Check sheet for the drawn part. Datum: minimum x, y, z corner. Units: mm. Give positions to 0.01 mm unless a question says otherwise; leave off trailing zeros. Loops run counter-clockwise (first coordinate to the right, second up) from the corner with the lowest first, then second, coordinate; pieces in that order, holes last. Notation, with made-up numbers: (76, -2) - (110, -2) arc R15 ccw to (110, 24) - close; hole circle Ø9 at (-7.5, 39). An arc over 180 degrees is marked (long way). Use one line per item in the form item = value.
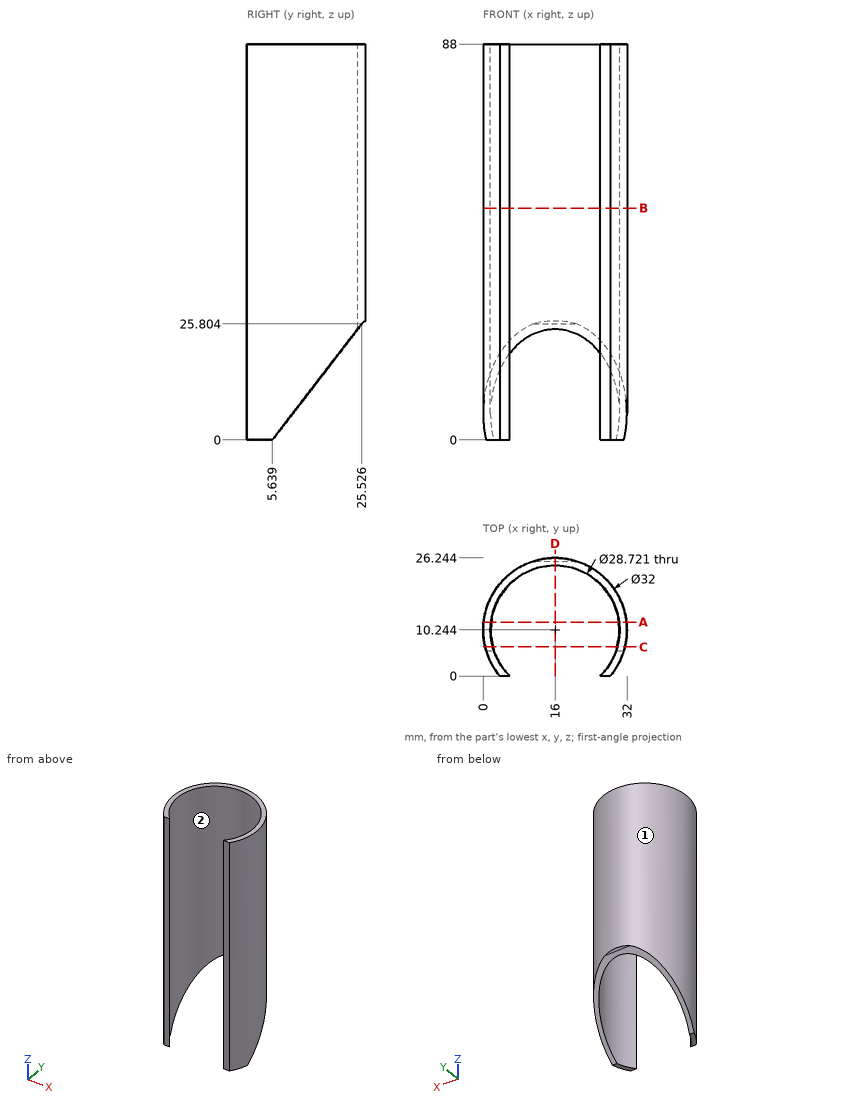
Item 1: Thickness scan on L1, parallel to X at y = 20.5, z = 43; L2, parallel to X at y = 9, z = 70.5; L3, parallel to Y at x = 16, z = 34.5. Record the ranges inside material, lowest first.
Answer block:
L1 = 3.72 to 5.95, 26.05 to 28.28
L2 = 0.05 to 1.69, 30.31 to 31.95
L3 = 24.6 to 26.24
Item 2: Section check D-D on x = 16. Record the boundary of the cut face in (y, z) (1 decimal), then the cut area to 3 significant figures.
Answer block:
outline = (24.6, 24.6) - (25.5, 25.8) - (26.2, 26.4) - (26.2, 88) - (24.6, 88) - close
area = 102 mm2
Item 3: Gauge pin test, flat ends, axial feed: P1, Ø6, axis at y = 12, z = 31, coming from the +X side; P2, Ø3, axis at x = 28, z = 46, coming from the +Y side (1 decimal). Record the tip position at first contact, or that the pin passes through.
Answer block:
P1 = 32
P2 = 22.3
Item 4: Section check A-A on y = 12. Record the boundary of the cut face in (x, z).
Answer block:
outline = (0.1, 8.25) - (1.75, 8.25) - (1.75, 88) - (0.1, 88) - close; (30.25, 8.25) - (31.9, 8.25) - (31.9, 88) - (30.25, 88) - close
Item 5: Section check B-B on z = 51.5. Record the boundary of the cut face in (x, y) (1 decimal), then the cut area to 3 significant figures.
Answer block:
outline = (3.7, 0) - (5.9, 0) arc R14.4 cw (long way) to (26.1, 0) - (28.3, 0) arc R16 ccw (long way) to start
area = 115 mm2
Item 6: Section check C-C on y = 6.5. Record the boundary of the cut face in (x, z) (1 decimal).
Answer block:
outline = (0.4, 1.1) - (2.1, 1.1) - (2.1, 88) - (0.4, 88) - close; (29.9, 1.1) - (31.6, 1.1) - (31.6, 88) - (29.9, 88) - close
Item 7: Mould release check, pull along Y, two halves, no side actions. Record for the marked faces 1 and 2: released by +Y, released by -Y, zero draft, split by the parting line, or undercut.
Answer block:
face_1 = split by the parting line
face_2 = undercut
